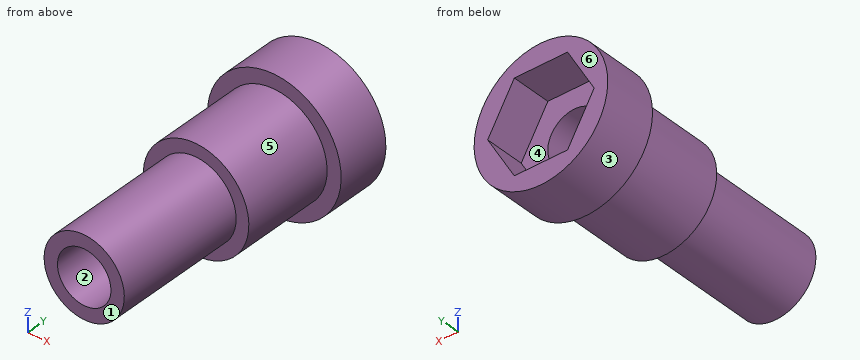
```python
from build123d import *

# Parameters (mm, degrees)
SKETCH1_R           = 3
SKETCH1_R_2         = 2
BOSS_EXTRUDE1_DEPTH = 18
BOSS_EXTRUDE3_START = -8
SKETCH2_R           = 3.95
SKETCH2_R_2         = 2
BOSS_EXTRUDE3_DEPTH = 7
SKETCH4_R           = 5
SKETCH4_R_2         = 2
BOSS_EXTRUDE4_DEPTH = 4
CUT_EXTRUDE1_DEPTH  = 3


with BuildPart() as part:
    # Sketch1 → Boss-Extrude1 (new body)
    with BuildSketch(Plane(origin=(0, 0, 0), x_dir=(1, 0, 0), z_dir=(0, 1, 0))):
        with Locations(Location((0, 0, 0), (0, 0, 270))):
            Circle(SKETCH1_R)
        with Locations(Location((0, 0, 0), (0, 0, 270))):
            Circle(SKETCH1_R_2, mode=Mode.SUBTRACT)
    extrude(amount=BOSS_EXTRUDE1_DEPTH)

    # Sketch2 → Boss-Extrude3 (add)
    with BuildSketch(Plane(origin=(0, 18, 0), x_dir=(1, 0, 0), z_dir=(0, 1, 0)).offset(BOSS_EXTRUDE3_START)):
        with Locations(Location((0, 0, 0), (0, 0, 270))):
            Circle(SKETCH2_R)
        with Locations(Location((0, 0, 0), (0, 0, 270))):
            Circle(SKETCH2_R_2, mode=Mode.SUBTRACT)
    extrude(amount=BOSS_EXTRUDE3_DEPTH)

    # Sketch4 → Boss-Extrude4 (add)
    with BuildSketch(Plane(origin=(0, 17, 0), x_dir=(1, 0, 0), z_dir=(0, 1, 0))):
        with Locations(Location((0, 0, 0), (0, 0, 270))):
            Circle(SKETCH4_R)
        with Locations(Location((0, 0, 0), (0, 0, 270))):
            Circle(SKETCH4_R_2, mode=Mode.SUBTRACT)
    extrude(amount=BOSS_EXTRUDE4_DEPTH)

    # Sketch5 → Cut-Extrude1 (cut)
    with BuildSketch(Plane(origin=(0, 21, 0), x_dir=(1, 0, 0), z_dir=(0, 1, 0))):
        Polygon((3.983716857, 0), (1.991858429, 3.45), (-1.991858429, 3.45), (-3.983716857, 0), (-1.991858429, -3.45), (1.991858429, -3.45), align=None)
    extrude(amount=-CUT_EXTRUDE1_DEPTH, mode=Mode.SUBTRACT)


solid = part.part
```
Model file for the job. Use its own axes, mm. Face numbers are marked on the shaded views. A direction names the side the tool comes from. Coordinates: 2 decimals unless noted, no trailing zeros. Loops run counter-clockwise (first coordinate to the right, second up) from the corner with the lowest first, then second, coordinate; pieces in that order, holes last. Notation, with made-up numbers: M 34,81.25 L 91,81.25 A19 cw 91,108.25 Z; hole C -24,67 d3. An arc over 180 degrees is marked long. Use CSV: the item, a comma, the result in double quotes. Start each with the question number.
1. Band-saw the part on A-A, the plane x = 0. List the corners of the cut face in (y, z).
2. Probe probe 1 along X at (y, z) = (14.25, 0); probe 2 along Z at (x, y) = (0, 9.5). List the from-to ranges inside material, lowest first. Write a range as [from, to].
3. Band-saw the part on D-D, the plane z = 2.25. List the corners of the cut face in (x, y), then the cut area to 3 significant figures.
4. Band-saw the part on B-B, the plane z = 0.5. List the corners of the cut face in (x, y), then the cut area to 3 significant figures.
5. Two-plate mould, pull along Z, no slides. Class the marked faces 1, 2 and 3: pulls with the +Z half, pulls with the -Z half, needs draft (parallel to the pull), parting line crosses it, or undercut.
6. Flat gauge pins, fed straight in: pin 1 (5.5 mm diameter, centred on x = 1, z = 0.5, fed in from +Y); pin 2 (1.5 mm diameter, centred on x = 2.5, y = 7, fed in from +Z); pin 3 (1 mm diameter, centred on y = 16, z = 3.5, fed in from -X); pin 4 (2 mm diameter, centred on x = -1, y = 13, fed in from +Z). Where does each tip first touch, or does it go through?
7. Tool access for the marked faces 4, 5 and 6: list every direction of +Z, -Z, +X, -X, +Y, -Y with a clear straight run to the whole face (end or side of a thin tool).
8. Band-saw the part on C-C, the plane y = 3.5. List the corners of the cut face in (x, z).
Entries:
1,outline,"M 0,-3 L 10,-3 L 10,-3.95 L 17,-3.95 L 17,-5 L 21,-5 L 21,-3.45 L 18,-3.45 L 18,-2 L 0,-2 Z; M 0,2 L 18,2 L 18,3.45 L 21,3.45 L 21,5 L 17,5 L 17,3.95 L 10,3.95 L 10,3 L 0,3 Z"
2,probe 1,"x = [-3.95, -2], [2, 3.95]"
2,probe 2,"z = [-3, -2], [2, 3]"
3,outline,"M -4.47,17 L -3.25,17 L -3.25,10 L -1.98,10 L -1.98,0 L 1.98,0 L 1.98,10 L 3.25,10 L 3.25,17 L 4.47,17 L 4.47,21 L 2.68,21 L 2.68,18 L -2.68,18 L -2.68,21 L -4.47,21 Z"
3,area,"105 mm2"
4,outline,"M -4.97,17 L -3.92,17 L -3.92,10 L -2.96,10 L -2.96,0 L -1.94,0 L -1.94,18 L -3.7,18 L -3.7,21 L -4.97,21 Z; M 1.94,0 L 2.96,0 L 2.96,10 L 3.92,10 L 3.92,17 L 4.97,17 L 4.97,21 L 3.7,21 L 3.7,18 L 1.94,18 Z"
4,area,"61.9 mm2"
5,face 1,"needs draft"
5,face 2,"undercut"
5,face 3,"parting line crosses it"
6,pin 1,"stops at y = 21"
6,pin 2,"stops at z = 2.44"
6,pin 3,"stops at x = -2.57"
6,pin 4,"stops at z = 3.95"
7,face 4,"+Y"
7,face 5,"-Y"
7,face 6,"+Z, -Z, +X, -X, +Y"
8,outline,"C 0,0 d6; hole C 0,0 d4"
